Part model, mm, in its own coordinate system. Face numbers are marked on the shaded views. Round coordinates to 2 decimals unless told otherwise and drop trailing zeros. Write each loop counter-clockwise with the first axis right and the second up, starting at its lowest first coordinate (ties: lowest second). Pieces come first, ordered by that corner, then holes.
1) Saw through at A-A on y = -8. Write the cut outline in (x, z).
2) Drill centre lines: L1, parallel to X at y = 19.5, z = 0; L2, parallel to Z at x = 0, y = 18; L3, parallel to Y at x = 11.25, z = 1.25. Where is each one in solid material? Low to high.
3) Pull direction Z, two halves, no side cores. Call the marked faces 1, 2, 3 and 4: +Z half, -Z half, draft (parallel to the pull), parting line (faces both ways), or undercut.
4) Flat gauge pins, fed straight in: pin 1 (1 mm diameter, centred on x = -6, z = -3, fed in from +Y); pin 2 (1.5 mm diameter, centred on y = 42.5, z = -4.5, fed in from -X). Where does each tip first touch, or does it go through?
```python
from build123d import *

# Parameters (mm, degrees)
SKETCH_1_R               = 12
EXTRUDE_1_DEPTH          = 50
SHELL_3_T                = -2
SKETCH_2_R               = 12
EXTRUDE_2_DEPTH          = 20
FILLET_1_R               = 2
SKETCH_5_R               = 0.25
CUT_EXTRUDE_1_DEPTH      = 54
PATTERN_CIRCULAR_1_COUNT = 50


with BuildPart() as part:
    # 草图1 → 凸台-拉伸1 (new body)
    with BuildSketch(Plane(origin=(0, 0, 0), x_dir=(1, 0, 0), z_dir=(0, 1, 0))):
        with Locations(Location((0, 0, 0), (0, 0, 270))):
            Circle(SKETCH_1_R)
    extrude(amount=EXTRUDE_1_DEPTH)

    # 抽壳3
    shell_3_openings = [part.faces().sort_by_distance(p)[0] for p in [
        (0, 50, 0),
    ]]
    offset(amount=SHELL_3_T, openings=shell_3_openings, kind=Kind.INTERSECTION)

    # 草图2 → 凸台-拉伸2 (add)
    with BuildSketch(Plane.XZ):
        with Locations(Location((0, 0, 0), (0, 0, 270))):
            Circle(SKETCH_2_R)
    extrude(amount=EXTRUDE_2_DEPTH)

    # 草图3 → 切除-旋转1 (revolve, cut)
    with BuildSketch(Plane.XY, mode=Mode.PRIVATE) as cut_revolve_1_sk:
        Polygon((11, -10), (11, -20), (12.743043998, -20), (12.743043998, -3), (10, -3), (10, -10), align=None)
    revolve(cut_revolve_1_sk.sketch.rotate(Axis((0, -0.535575004, 0), (0, -1, 0)), 180), axis=Axis((0, -0.535575004, 0), (0, -1, 0)), mode=Mode.SUBTRACT)

    # 圆角1
    fillet_1_edges = [part.edges().sort_by_distance(p)[0] for p in [
        (11, -20, 0),
    ]]
    fillet(fillet_1_edges, radius=FILLET_1_R)

    # 草图5 → 切除-拉伸1 (cut)
    with BuildSketch(Plane(origin=(0, 50, 0), x_dir=(1, 0, 0), z_dir=(0, 1, 0))):
        with Locations((12, 0)):
            Circle(SKETCH_5_R)
    cut_extrude_1 = extrude(amount=-CUT_EXTRUDE_1_DEPTH, mode=Mode.SUBTRACT)

    # 阵列(圆周)1: 切除-拉伸1 ×50 about axis, 6 skipped
    pattern_circular_1_axis = Axis((0, 0, 0), (0, -1, 0))
    add([cut_extrude_1.rotate(pattern_circular_1_axis, i * 360 / PATTERN_CIRCULAR_1_COUNT) for i in range(1, PATTERN_CIRCULAR_1_COUNT) if i not in (36, 37, 38, 39, 40, 41)], mode=Mode.SUBTRACT)


solid = part.part
```
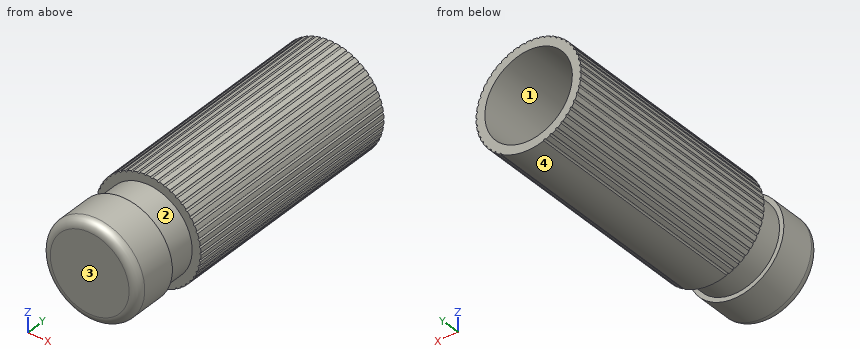
Completed:
1. outline: circle Ø20 at (0, 0)
2. L1: x = -11.75 to -10, 10 to 11.75
2. L2: z = -12 to -10, 10 to 12
2. L3: y = -3 to 50
3. face 1: undercut
3. face 2: parting line
3. face 3: draft
3. face 4: -Z half
4. pin 1: stops at y = 2
4. pin 2: stops at x = -11.4
